Geometry: final body of the model. Coordinates: model frame, mm. A direction names the side the tool comes from. Give positions to 0.01 mm unless a question says otherwise; leave off trailing zeros. Write each loop counter-clockwise with the first axis right and the second up, starting at its lowest first coordinate (ties: lowest second). Pieces come first, ordered by that corner, then holes. Notation, with made-up numbers: (83, 58) -> (135, 58) arc R21 cw to (135, 93) -> close; hole circle Ø3 at (-8, 75.25). An arc over 180 degrees is marked (long way). Answer as a JSON object with one key per item and string values. Group by question number.
(1) Material intervals for probe 1 along Y at (x, z) = (1.15, 96.25); probe 2 along Z at (x, y) = (0.7, 5.35); probe 3 along Y at (x, z) = (0.75, 96), sorted ascending.
(2) Section query A-A on z = 99. Output: boundary loops of the cut face in (x, y).
(3) Section query C-C on x = 0.45. Output: boundary loops of the cut face in (y, z), plus the area to 3 significant figures.
(4) Contact query for a flat-ended pin moving along its axis: pin 1 Ø2 at (y, z) = (4, 101) entering from -X. Output: stop coordinate, or through.
(5) Draft query along Z for faces 4 (the face through (0.74, 5.093, 99.371)), 5 (the face through (0.74, 8.7, 95.46)), 6 (the face through (0.74, 3.46, 98.28)). Return one class per face: +Z half, -Z half, draft (parallel to the pull), parting line (faces both ways), or undercut.
(6) Set-up query: faces 1 (the face through (1.5, 6, 98)), 2 (the face through (0.74, 4.32, 98.9)), 3 (the face through (0.74, 4.956, 100.257)). Return all of +Z, -Z, +X, -X, +Y, -Y with unobstructed straight access to the full face (end or side cutting, diameter ignored); none if empty.
(7) Section query B-B on y = 5.1. Output: boundary loops of the cut face in (x, z).
(8) Section query D-D on y = 6.05. Output: boundary loops of the cut face in (x, z), plus the area to 3 significant figures.
from build123d import *

# Parameters (mm, degrees)
SKETCH1_R           = 0.5
BOSS_EXTRUDE1_DEPTH = 1.5


with BuildPart() as part:
    # Sketch1 → Boss-Extrude1 (new body)
    with BuildSketch(Plane(origin=(0, 0, 0), x_dir=(0, 0, -1), z_dir=(1, 0, 0))):
        with BuildLine():
            Line((-97.427906133, 3.051254101), (-95.263862375, 7.558682926))
            ThreePointArc((-95.263862375, 7.558682926), (-95.469674877, 8.709850021), (-96.626851501, 8.878630138))
            Line((-96.626851501, 8.878630138), (-101.727897648, 6.224985812))
            Line((-101.727897648, 6.224985812), (-102.1607064, 5.323500047))
            Line((-102.1607064, 5.323500047), (-100.47042059, 4.511983637))
            Line((-100.47042059, 4.511983637), (-100.037611839, 5.413469402))
            Line((-100.037611839, 5.413469402), (-98.685383191, 4.764256275))
            Line((-98.685383191, 4.764256275), (-99.118191943, 3.86277051))
            Line((-99.118191943, 3.86277051), (-97.427906133, 3.051254101))
        make_face()
        with Locations((-96.16534814, 7.991491677)):
            Circle(SKETCH1_R, mode=Mode.SUBTRACT)
    extrude(amount=BOSS_EXTRUDE1_DEPTH)


solid = part.part
Answer list:
{
 "1": {"probe 1": "5.5 to 7.5, 8.48 to 8.99", "probe 2": "96.32 to 99.91, 100.07 to 102.15", "probe 3": "6.03 to 7.52, 8.46 to 8.98"},
 "2": {"outline": "(0, 3.81) -> (1.5, 3.81) -> (1.5, 4.11) -> (0, 4.11) -> close; (0, 4.92) -> (1.5, 4.92) -> (1.5, 7.64) -> (0, 7.64) -> close"},
 "3": {"outline": "(3.05, 97.43) -> (7.56, 95.26) arc R1 ccw to (8.88, 96.63) -> (6.22, 101.73) -> (5.32, 102.16) -> (4.51, 100.47) -> (5.41, 100.04) -> (4.76, 98.69) -> (3.86, 99.12) -> close; hole circle Ø1 at (7.99, 96.17)", "area": "19.6 mm2"},
 "4": {"pin 1": "x = 0"},
 "5": {"face 4": "undercut", "face 5": "parting line", "face 6": "+Z half"},
 "6": {"face 1": "+Z, -Z, +X, +Y, -Y", "face 2": "+X, -X", "face 3": "+X, -X, -Y"},
 "7": {"outline": "(0, 96.44) -> (1.5, 96.44) -> (1.5, 99.38) -> (0, 99.38) -> close; (0, 100.19) -> (1.5, 100.19) -> (1.5, 101.7) -> (0, 101.7) -> close"},
 "8": {"outline": "(0, 95.99) -> (1.5, 95.99) -> (1.5, 101.81) -> (0, 101.81) -> close", "area": "8.74 mm2"}
}
